Job drawing, mm, ordinate dimensions from the low corner. One solid piece. A direction names the side the tool comes from. Give positions to 0.01 mm unless a question says otherwise; leave off trailing zeros. Order: outer loops, then holes, each group sorted by start corner. A loop starts at its lowest first (then second) coordinate and runs counter-clockwise, first axis right, second up.
1. Drop flat-ended pins along their axis: pin 1 Ø1.5 at (x, y) = (6, 4.5) entering from -Z (1 decimal); pin 2 Ø3 at (x, z) = (7, 4.5) entering from -Y; pin 3 Ø0.8 at (x, z) = (1, 3.5) entering from +Y. Give the stop position or say it passes through.
2. Probe line 1 (Y direction, x = 1, z = 4.1); line 2 (Y direction, x = 1, z = 2.15) (1 decimal); line 3 (Z direction, x = 5.5, y = 3.55). List the from-to ranges inside material, lowest first.
3. Mould opens along Y. For the marked faces 1, 2 and 3 say: +Y half, -Y half, draft (parallel to the pull), parting line (faces both ways), or undercut.
4. Which spindle directions (+Z, -Z, +X, -X, +Y, -Y) get a long thin tool onto all of the face, cutting with end or side? Do the marked faces 4 and 5. Say none if no direction does.
5. Slice it at A-A on x = 8.25. List the corners of the cut face in (y, z), and give its area (3 significant figures).
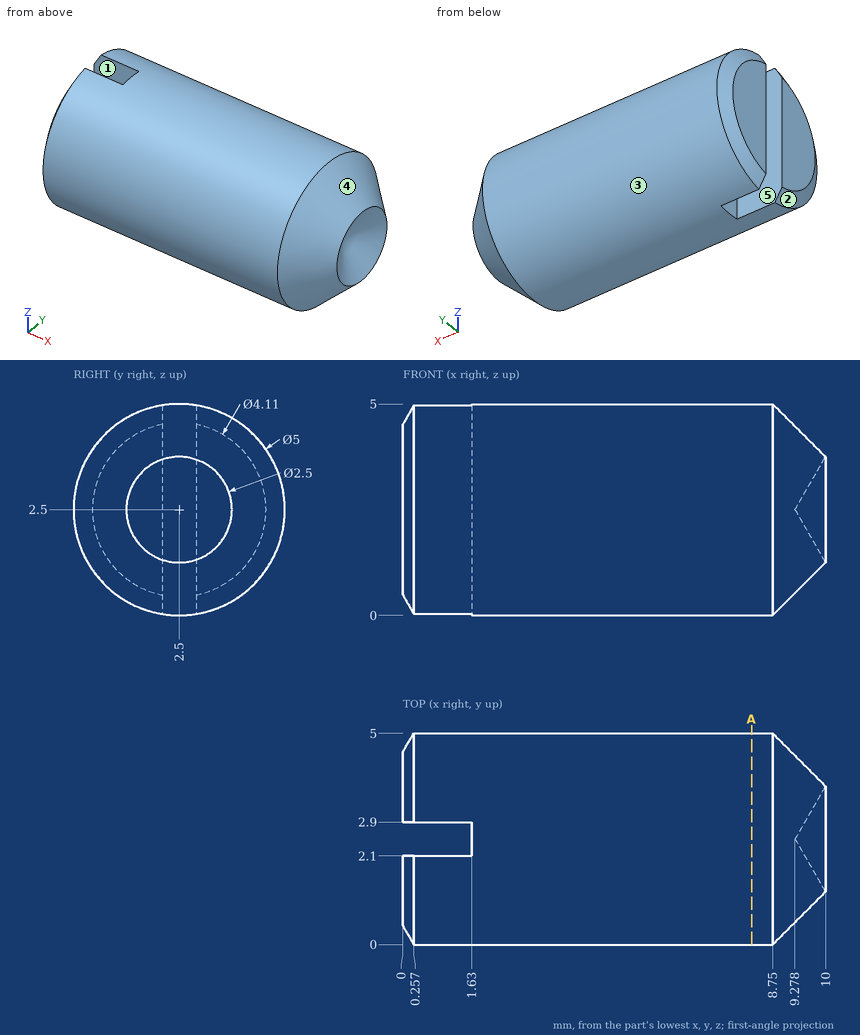
Data:
1. pin 1: stops at z = 0.3
1. pin 2: stops at y = 0.05
1. pin 3: stops at y = 4.93
2. line 1: y = 0.58 to 2.1, 2.9 to 4.42
2. line 2: y = 0 to 2.1, 2.9 to 5
2. line 3: z = 0.23 to 4.77
3. face 1: undercut
3. face 2: -Y half
3. face 3: parting line
4. face 4: +X
4. face 5: +Z, -Z, -X
5. outline: circle Ø5 at (2.5, 2.5)
5. area: 19.6 mm2
